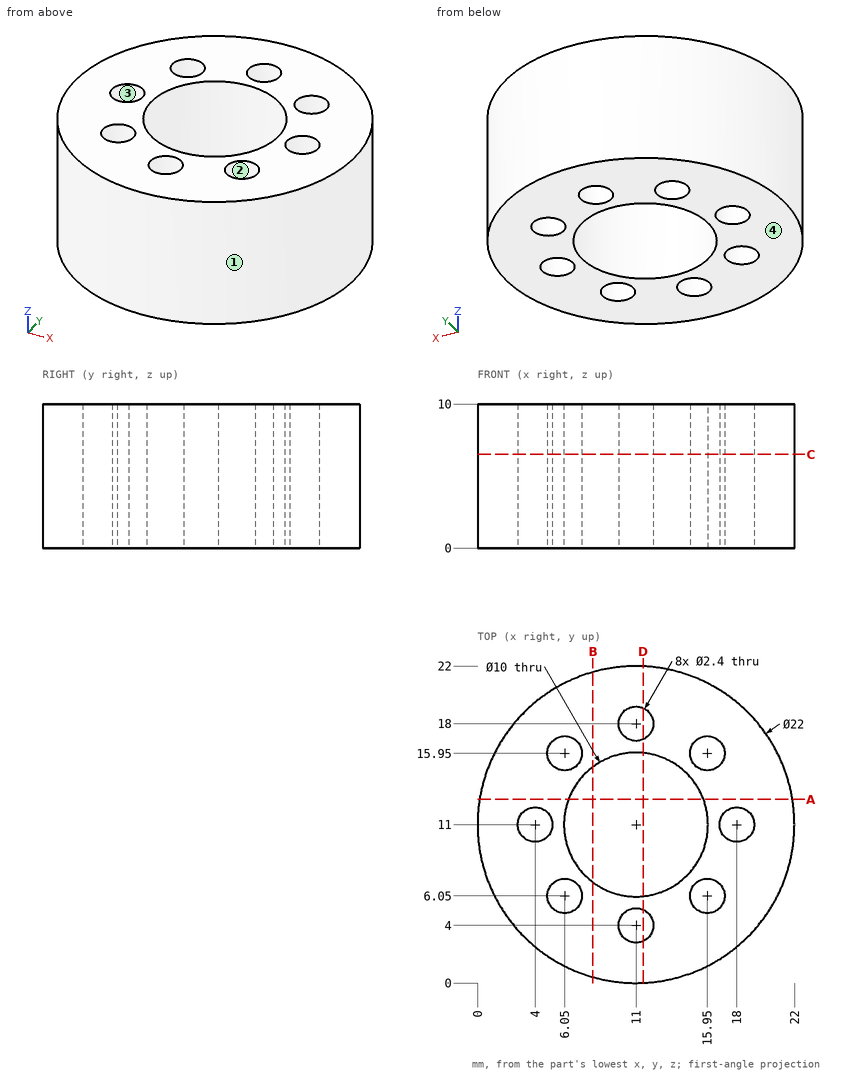
Geometry check sheet. Reference: drawing and pictorial views, mm from the part's lowest x, y, z. Give positions to 0.01 mm unless a question says otherwise; leave off trailing zeros. Write each loop counter-clockwise with the first axis right and the second up, starting at its lowest first coordinate (ties: lowest second). Pieces come first, ordered by that corner, then holes. Notation, with made-up numbers: M 24.5,87.25 L 71.5,87.25 A18 ccw 71.5,95.25 Z; hole C 11.5,68.5 d6. An arc over 180 degrees is marked long. Put each result on its own line as item: value. Start each with the question number.
1. Scan lines: line 1 along X through (y, z) = (11.75, 3.5) (1 decimal); line 2 along X through (y, z) = (6.75, 7.25) (1 decimal); line 3 along X through (y, z) = (13.5, 6.25). Record each from-to range of solid material in increasing order. Write a range as [from, to].
2. Section check D-D (x = 11.5). Record the cut outline in (y, z) (1 decimal).
3. Section check B-B (x = 8). Record the cut outline in (y, z), and give its area (3 significant figures).
4. Section check C-C (z = 6.5). Give the number of separate pieces and of enclosed holes in the cut face, and give its area (3 significant figures).
5. Go/stop test with flat-tipped pins: pin 1 Ø1.9 at (x, y) = (4, 11) entering from +Z; pin 2 Ø2 at (x, z) = (14.5, 3) entering from +Y; pin 3 Ø6 at (y, z) = (6, 5) entering from +X; pin 4 Ø4 at (x, z) = (6.5, 6.5) entering from -Y. Record where each tip stops, or that it passes through.
6. Section check A-A (y = 12.75). Record the cut outline in (x, z).
7. Draft check along Y on the marked faces 1, 2, 3 and 4. Enter one of: +Y half, -Y half, draft (parallel to the pull), parting line (faces both ways), or undercut.
Answer list:
1. line 1: [0, 3.1], [4.9, 6.1], [15.9, 17.1], [18.9, 22]
1. line 2: [0.9, 5.1], [7, 8.4], [13.6, 15], [16.9, 21.1]
1. line 3: [0.29, 6.67], [15.33, 21.71]
2. outline: M 0,0 L 2.9,0 L 2.9,10 L 0,10 Z; M 5.1,0 L 6,0 L 6,10 L 5.1,10 Z; M 16,0 L 16.9,0 L 16.9,10 L 16,10 Z; M 19.1,0 L 22,0 L 22,10 L 19.1,10 Z
3. outline: M 0.42,0 L 7,0 L 7,10 L 0.42,10 Z; M 15,0 L 21.58,0 L 21.58,10 L 15,10 Z
3. area: 132 mm2
4. separate pieces: 1
4. enclosed holes: 9
4. area: 265 mm2
5. pin 1: through
5. pin 2: y = 21.71
5. pin 3: x = 21.82
5. pin 4: y = 0.29
6. outline: M 0.14,0 L 6.32,0 L 6.32,10 L 0.14,10 Z; M 15.68,0 L 21.86,0 L 21.86,10 L 15.68,10 Z
7. face 1: parting line
7. face 2: undercut
7. face 3: undercut
7. face 4: draft
